Autodesk Inventor part; units mm, degrees
ref_plane "YZ Plane" through (0, 0, 0) normal (1, 0, 0) x (0, 1, 0)
ref_plane "XZ Plane" through (0, 0, 0) normal (0, 1, 0) x (-1, 0, 0)
ref_plane "XY Plane" through (0, 0, 0) normal (0, 0, 1) x (1, 0, 0)
sketch "Sketch1" plane through (0, 0, 0) normal (0, 1, 0) x (-1, 0, 0)
  circle A0 centre (0, 0) radius 2.8702
  dimension "d0" = 5.7404
extrude "Extrusion1" add sketch "Sketch1" along normal blind 3.4036
sketch "Sketch2" plane through (0, 3.4036, 0) normal (0, 1, 0) x (1, 0, 0)
  circle A0 centre (0, 0) radius 4.445
  line L0 (0, 0) -> (0, 10)
  circle A1 centre (0, 10) radius 1
  circle A2 centre (0, 10) radius 2.54
  line L1 (-4.3636, 0.8468) -> (-2.4935, 10.4839)
  line L2 (4.3636, 0.8468) -> (2.4935, 10.4839)
  dimension "d3" = 8.89
  dimension "d4" = 10
  dimension "d5" = 2
  dimension "d6" = 5.08
extrude "Extrusion2" add sketch "Sketch2" along normal blind 1.905
sketch "Sketch3" plane through (0, 5.3086, 0) normal (0, 1, 0) x (1, 0, 0)
  circle A0 centre (0, 0) radius 1.27
  dimension "d9" = 2.54
extrude "Extrusion3" cut sketch "Sketch3" against normal through all
sketch "Sketch4" plane through (0, 5.3086, 0) normal (0, 1, 0) x (1, 0, 0)
  circle A0 centre (0, 0) radius 3.175
  dimension "d12" = 6.35
extrude "Extrusion4" cut sketch "Sketch4" against normal blind 1.016
sketch "Sketch5" plane through (0, 0, 0) normal (0, -1, 0) x (1, 0, 0)
  circle A0 centre (0, 0) radius 4.445
  circle A1 centre (0, 0) radius 2.8702
  arc A2 (4.3636, -0.8468) -> (-4.3636, -0.8468) centre (0, 0) ccw
  dimension "d21" = 8.89
extrude "Extrusion6" add sketch "Sketch5" against normal up to surface (3.4036 mm away)
extrude "Extrusion7" cut sketch "Sketch5" against normal blind 3.4036 contours A1
properties part number "ServoHorn10mmPitch" material "ABS Plastic"
Work out the finished part from the listing and answer in its coordinate system (mm). A direction names the side the tool comes from. Give positions to 0.01 mm unless a question says otherwise; leave off trailing zeros. Order: outer loops, then holes, each group sorted by start corner. A loop starts at its lowest first (then second) coordinate and runs counter-clockwise, first axis right, second up. Notation, with made-up numbers: (42, 20.25) - (83, 20.25) arc R11 cw to (83, 38.25) - close; hole circle Ø11 at (23, 72). An arc over 180 degrees is marked (long way). Answer as CSV lines item,"result". Start each with the question number.
Q1. The mould has two halves that part along X. Classify faces 1 (the face through (0.041, 2.027, 4.445)), 2 (the face through (3, 0, -1)), 3 (the face through (-0.17, 3.85, -1.26)): +X half, -X half, draft (parallel to the pull), parting line (faces both ways), or undercut.
Q2. The part is cut by section A-A (x = 0). Write down the section's boundary in (y, z) (3 decimals), then the cut area to 3 significant figures.
Q3. The part is cut by section B-B (z = -10). Write down the section's boundary in (x, y).
Q4. For faces 4 (the face through (-0.69, 4.81, 3.1)), 5 (the face through (3.44, 4.34, -5.6)), 6 (the face through (-2.278, 1.678, -1.746)), determine the directions among +Z, -Z, +X, -X, +Y, -Y from which every point of the face is accessible in a straight line to the end or side of a thin tool.
Q5. The part is cut by section D-D (y = 0.55). Write down the section's boundary in (x, z) (3 decimals).
Q6. The part is cut by section C-C (y = 4.85). Give the number of separate pieces and of enclosed holes in the cut face, then the cut area to 3 significant figures.
Q7. Find the intervals of material crossed by L1, parallel to Z at x = 0, y = 3.85 (3 decimals); L2, parallel to Z at x = 0, y = 5.05 (3 decimals); L3, parallel to Z at x = 0, y = 2 (3 decimals), in increasing order. Write a range as [from, to].
Q8. Given pin 1 Ø1.5 at (x, y) = (-2.5, 2) entering from +Z; pin 2 Ø3 at (y, z) = (4, -3) entering from +X; pin 3 Ø2.5 at (x, z) = (0, -10) entering from -Y; pin 4 Ø2 at (x, z) = (0, 0) entering from +Y, each flat-ended and moving along its own axis, determine where each tip first touches the part or whether it passes through.
Check result:
1,face 1,"parting line"
1,face 2,"draft"
1,face 3,"undercut"
2,outline,"(0, -4.445) - (3.404, -4.445) - (3.404, -9) - (5.309, -9) - (5.309, -3.175) - (4.293, -3.175) - (4.293, -1.27) - (3.404, -1.27) - (3.404, -2.87) - (0, -2.87) - close; (0, 2.87) - (3.404, 2.87) - (3.404, 1.27) - (4.293, 1.27) - (4.293, 3.175) - (5.309, 3.175) - (5.309, 4.445) - (0, 4.445) - close; (3.404, -12.54) - (5.309, -12.54) - (5.309, -11) - (3.404, -11) - close"
2,area,"30.6 mm²"
3,outline,"(-2.59, 3.4) - (-1, 3.4) - (-1, 5.31) - (-2.59, 5.31) - close; (1, 3.4) - (2.59, 3.4) - (2.59, 5.31) - (1, 5.31) - close"
4,face 4,"+Y"
4,face 5,"-Z, +X, +Y, -Y"
4,face 6,"-Y"
5,outline,"circle Ø8.89 at (0, 0); hole circle Ø5.74 at (0, 0)"
6,separate pieces,"1"
6,enclosed holes,"2"
6,area,"77.5 mm²"
7,L1,"z = [-12.54, -11], [-9, -1.27], [1.27, 4.445]"
7,L2,"z = [-12.54, -11], [-9, -3.175], [3.175, 4.445]"
7,L3,"z = [-4.445, -2.87], [2.87, 4.445]"
8,pin 1,"stops at z = 4.09"
8,pin 2,"stops at x = 4.24"
8,pin 3,"stops at y = 3.4"
8,pin 4,"passes through"
